```python
from build123d import *

# Parameters (mm, degrees)
BOSS_EXTRUDE1_DEPTH = 0.25


with BuildPart() as part:
    # Sketch1 → Boss-Extrude1 (new, symmetric)
    with BuildSketch(Plane(origin=(0, 0, 0), x_dir=(1, 0, 0), z_dir=(0, 1, 0))):
        with BuildLine():
            Line((-22.5, 57.39480496), (22.5, 57.39480496))
            Line((22.5, 57.39480496), (22.5, 157.39480496))
            Line((22.5, 157.39480496), (90.871933013, 157.39480496))
            Line((90.871933013, 157.39480496), (91, 157.616623489))
            ThreePointArc((91, 157.616623489), (0, 182), (-91, 157.616623489))
            Line((-91, 157.616623489), (-90.871933013, 157.39480496))
            Line((-90.871933013, 157.39480496), (-22.5, 157.39480496))
            Line((-22.5, 157.39480496), (-22.5, 57.39480496))
        make_face()
        with BuildLine():
            Line((-16.75, 85.19480496), (-16.75, 65.19480496))
            ThreePointArc((-16.75, 65.19480496), (-12.5, 60.94480496), (-8.25, 65.19480496))
            Line((-8.25, 65.19480496), (-8.25, 85.19480496))
            ThreePointArc((-8.25, 85.19480496), (-12.5, 89.44480496), (-16.75, 85.19480496))
        make_face(mode=Mode.SUBTRACT)
        with BuildLine():
            Line((16.75, 85.19480496), (16.75, 65.19480496))
            ThreePointArc((16.75, 65.19480496), (12.5, 60.94480496), (8.25, 65.19480496))
            Line((8.25, 65.19480496), (8.25, 85.19480496))
            ThreePointArc((8.25, 85.19480496), (12.5, 89.44480496), (16.75, 85.19480496))
        make_face(mode=Mode.SUBTRACT)
    extrude(amount=BOSS_EXTRUDE1_DEPTH, both=True)


solid = part.part
```
Geometry: final body of the model. Coordinates: model frame, mm. A direction names the side the tool comes from. Round coordinates to 2 decimals unless told otherwise and drop trailing zeros. Order: outer loops, then holes, each group sorted by start corner. A loop starts at its lowest first (then second) coordinate and runs counter-clockwise, first axis right, second up. Notation, with made-up numbers: M 51.5,27.25 L 65.5,27.25 A15 ccw 65.5,55.25 Z; hole C 69.5,-14.75 d8. An arc over 180 degrees is marked long. Use one line per item in the form item = value. Start each with the question number.
Q1. Cut plane C-C (z = -138.5). Return loops of the section in (x, y), and give its area (3 significant figures).
Q2. Cut plane D-D (x = 40). Return loops of the section in (y, z).
Q3. Cut plane B-B (x = 12.5). Return loops of the section in (y, z), and give its area (3 significant figures).
Q4. Cut plane A-A (y = 0.1). Return loops of the section in (x, z), and give its area (3 significant figures).
Q5. Access query for faces 4 (the face through (-12.593, 0.004, -60.946)), 5 (the face through (-1, -0.25, -134)). Directions: +Z, -Z, +X, -X, +Y, -Y. A direction counts if a zero-diameter tool reaches every point of the face in a straight line with its end or side. Return the directions, or none.
Q6. Mould query, pull axis X, two halves, no side actions, for faces 1 (the face through (-1, 0.25, -134)), 2 (the face through (1.334, 0.004, -181.995)), 3 (the face through (12.593, 0.004, -60.946)). Classes: +X half, -X half, draft (parallel to the pull), parting line (faces both ways), or undercut.
Q7. Material intervals for line 1 (X direction, y = 0.2, z = -87); line 2 (X direction, y = -0.15, z = -107); line 3 (Z direction, x = -12, y = -0.05), sorted ascending. Write a range as [from, to].
Geometry results:
q1.outline = M -22.5,-0.25 L 22.5,-0.25 L 22.5,0.25 L -22.5,0.25 Z
q1.area = 22.5 mm^2
q2.outline = M -0.25,-177.55 L 0.25,-177.55 L 0.25,-157.39 L -0.25,-157.39 Z
q3.outline = M -0.25,-181.57 L 0.25,-181.57 L 0.25,-89.44 L -0.25,-89.44 Z; M -0.25,-60.94 L 0.25,-60.94 L 0.25,-57.39 L -0.25,-57.39 Z
q3.area = 47.8 mm^2
q4.outline = M -91,-157.62 A182 ccw 91,-157.62 L 90.87,-157.39 L 22.5,-157.39 L 22.5,-57.39 L -22.5,-57.39 L -22.5,-157.39 L -90.87,-157.39 Z; hole M -16.75,-85.19 A4.25 ccw -8.25,-85.19 L -8.25,-65.19 A4.25 ccw -16.75,-65.19 Z; hole M 8.25,-85.19 A4.25 ccw 16.75,-85.19 L 16.75,-65.19 A4.25 ccw 8.25,-65.19 Z
q4.area = 7,090 mm^2
q5.face_4 = +Y, -Y
q5.face_5 = +Z, -Z, +X, -X, -Y
q6.face_1 = draft
q6.face_2 = parting line
q6.face_3 = undercut
q7.line_1 = [-22.5, -16.35], [-8.65, 8.65], [16.35, 22.5]
q7.line_2 = [-22.5, 22.5]
q7.line_3 = [-181.6, -89.42], [-60.97, -57.39]
